```python
from build123d import *

# Parameters (mm, degrees)
F1_DEPTH = 1
F2_W     = 19.8857705285
F2_H     = 1
F3_DEPTH = 12
F4_W     = 8
F4_H     = 26
F5_DEPTH = 1.001
F6_R     = 1.5
F7_DEPTH = 1.001
F8_R     = 5


with BuildPart() as f1:
    # F0 (on Top) → F1 (new body)
    with BuildSketch(Plane.XY):
        with BuildLine():
            Line((-9, 19.25), (-9, -19.25))
            ThreePointArc((-9, -19.25), (21.25, 0), (-9, 19.25))
        make_face()
    extrude(amount=F1_DEPTH)

    # F2 (on face) → F3 (join)
    with BuildSketch(Plane.XY.offset(1)):
        with Locations((0.9428852643, -17.75)):
            Rectangle(F2_W, F2_H)
    extrude(amount=F3_DEPTH)

    # F4 (on face) → F5 (cut, through all)
    with BuildSketch(Plane.XY.offset(1)):
        with Locations((-2.5, -0.25)):
            Rectangle(F4_W, F4_H)
        with Locations((11, -0.25)):
            Rectangle(F4_W, F4_H)
    extrude(amount=-F5_DEPTH, mode=Mode.SUBTRACT)

    # F6 (on face) → F7 (cut, through all)
    with BuildSketch(Plane.XY.offset(1)):
        with Locations((0, -20.8)):
            Circle(F6_R)
        with Locations((20.8, 0)):
            Circle(F6_R)
        with Locations((0, 20.8)):
            Circle(F6_R)
        with Locations((-20.8, 0)):
            Circle(F6_R)
    extrude(amount=-F7_DEPTH, mode=Mode.SUBTRACT)

    # F8
    f8_edges = [f1.edges().sort_by_distance(p)[0] for p in [
        (1.445467, -21.200781, 0.5),
        (-1.445467, -21.200781, 0.5),
        (21.200781, 1.445467, 0.5),
        (21.200781, -1.445467, 0.5),
        (1.445467, 21.200781, 0.5),
        (-1.445467, 21.200781, 0.5),
    ]]
    fillet(f8_edges, radius=F8_R)


solid = f1.part
```
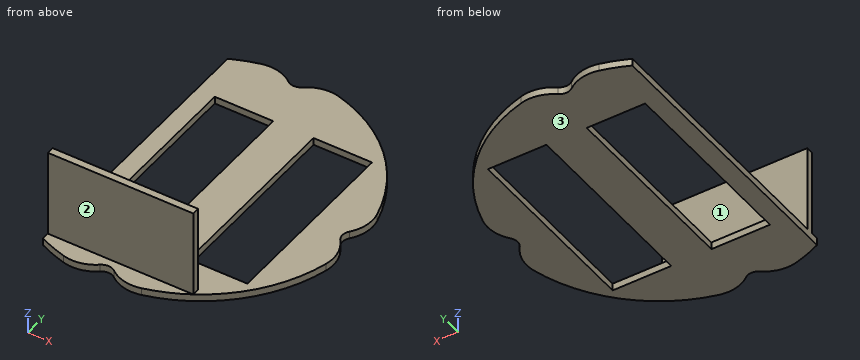
Work out the finished part from the listing and answer in its coordinate system (mm). Face numbers are marked on the shaded views. A direction names the side the tool comes from. Give positions to 0.01 mm unless a question says otherwise; leave off trailing zeros. Order: outer loops, then holes, each group sorted by start corner. A loop starts at its lowest first (then second) coordinate and runs counter-clockwise, first axis right, second up.
1. Section A-A, the plane x = 0 is taken. Determine the outline of the cut face in (y, z).
Result sheet:
outline: (-19.3, 0) - (-13.25, 0) - (-13.25, 1) - (-17.25, 1) - (-17.25, 13) - (-18.25, 13) - (-18.25, 1) - (-19.3, 1) - close; (12.75, 0) - (19.3, 0) - (19.3, 1) - (12.75, 1) - close
2. Section C-C, the plane x = 9.25 is taken. Determine the outline of the cut face in (y, z), and give its area (3 significant figures).
Result sheet:
outline: (-19.13, 0) - (-13.25, 0) - (-13.25, 1) - (-17.25, 1) - (-17.25, 13) - (-18.25, 13) - (-18.25, 1) - (-19.13, 1) - close; (12.75, 0) - (19.13, 0) - (19.13, 1) - (12.75, 1) - close
area: 24.3 mm2
3. For the marked faces 1, 2 and 3, determine the directions among +Z, -Z, +X, -X, +Y, -Y from which every point of the face is accessible in a straight line to the end or side of a thin tool.
Result sheet:
face 1: +Z, +X, -X, +Y
face 2: +Z, +X, -X, -Y
face 3: -Z, +X, -X, +Y, -Y
4. Section B-B, the plane y = 8 is taken. Determine the outline of the cut face in (x, z).
Result sheet:
outline: (-9, 0) - (-6.5, 0) - (-6.5, 1) - (-9, 1) - close; (1.5, 0) - (7, 0) - (7, 1) - (1.5, 1) - close; (15, 0) - (19.69, 0) - (19.69, 1) - (15, 1) - close
5. Straight lines are drawn through the part: L1, parallel to Y at x = -6.5, z = 9.5; L2, parallel to Z at x = 19, y = 2.5; L3, parallel to X at y = -15.5, z = 0.5. For each, find the intervals that lie inside material, in ascending order.
Result sheet:
L1: y = -18.25 to -17.25
L2: z = 0 to 1
L3: x = -9 to 14.54
6. Each of these flat-tipped pins is pushed along its axis until it touches: P1, Ø0.5, axis at y = 3, z = 0.5, coming from the +X side; P2, Ø15, axis at x = 1, y = 0, coming from the +Z side; P3, Ø6, axis at x = -2, z = 11, coming from the -Y side; P4, Ø6, axis at y = 15, z = 4.5, coming from the +X side. Where does it stop, or does it pass through?
Result sheet:
P1: stops at x = 20.66
P2: stops at z = 1
P3: stops at y = -18.25
P4: passes through
7. Section D-D, the plane z = 1.5 is taken. Determine the outline of the cut face in (x, y).
Result sheet:
outline: (-9, -18.25) - (10.89, -18.25) - (10.89, -17.25) - (-9, -17.25) - close
